Can you work these out from the model? Positions are in its coordinate system, mm. Face numbers are marked on the shaded views. A direction names the side the tool comes from. Give positions to 0.01 mm unless a question says otherwise; leave off trailing zeros. Write each loop counter-clockwise with the first axis right and the second up, starting at its lowest first coordinate (ties: lowest second). Pieces come first, ordered by that corner, then holes.
Autodesk Inventor part; units mm, degrees
ref_plane "YZ Plane" through (0, 0, 0) normal (1, 0, 0) x (0, 1, 0)
ref_plane "XZ Plane" through (0, 0, 0) normal (0, 1, 0) x (-1, 0, 0)
ref_plane "XY Plane" through (0, 0, 0) normal (0, 0, 1) x (1, 0, 0)
sketch "Skizze1" plane through (0, 0, 0) normal (0, 1, 0) x (-1, 0, 0)
  arc A0 (-8, 0) -> (8, 0) centre (0, 0) ccw
  line L0 (8, 0) -> (8, 11)
  line L1 (8, 17) -> (-8, 17)
  line L2 (-8, 17) -> (-8, 0)
  line L3 (8, 17) -> (19, 17)
  line L4 (19, 17) -> (19, 11)
  line L5 (19, 11) -> (8, 11)
  dimension "d0" = 16
  dimension "d1" = 16
  dimension "d2" = 6
  dimension "d3" = 19
  dimension "d4" = 11
  dimension "d5" = 17
extrude "Extrusion1" add sketch "Skizze1" along normal blind 50
sketch "Skizze2" plane through (0, 50, 0) normal (0, 1, 0) x (1, 0, 0)
  arc A0 (8, 0) -> (-8, 0) centre (0, 0) ccw
hole "Bohrung1" at (0, 50, 0) direction (0, -1, 0) diameter 6 end through all
sketch "Skizze3" plane through (-19, 0, 11) normal (-1, 0, 0) x (0, 0, 1)
  line L0 (0, 0) -> (0, 50)
  line L1 (0, 31) -> (-11, 31)
  arc A0 (-11, 31) -> (-11, 19) centre (-11, 25) ccw
  line L2 (-11, 19) -> (0, 19)
  line L3 (0, 31) -> (0, 19)
  point P0 (-11, 0)
  point P1 (0, 25)
  dimension "d15" = 6
extrude "Extrusion2" add sketch "Skizze3" against normal up to surface (11 mm away)
sketch "Skizze4" plane through (-19, 0, 11) normal (-1, 0, 0) x (0, 0, 1)
  arc A0 (-11, 31) -> (-11, 19) centre (-11, 25) ccw
  point P0 (-11, 0)
hole "Bohrung2" at (-19, 25, 0) direction (1, 0, 0) diameter 9 depth 11
sketch "Skizze5" plane through (-8, 50, 11) normal (0, 0, -1) x (-1, 0, 0)
  line L0 (11, -19) -> (11, 0)
  line L1 (11, -31) -> (11, -19)
  point P0 (-8, -50)
  point P1 (4.5, -12.5)
  point P2 (4.5, -37.5)
  point P3 (11, -25)
  dimension "d32" = 6.5
  dimension "d33" = 12.5
  dimension "d34" = 25
hole "Bohrung3" at (-12.5, 37.5, 11) at (-12.5, 12.5, 11) direction (0, 0, 1) diameter 4.134 end through all
properties part number "103"
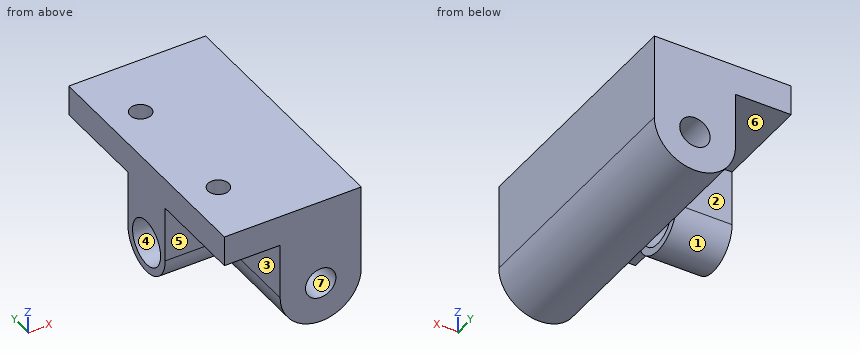
(1) Imagine slicing it at C-C, the plane z = 15.25. Write out the boundary of the cut face in (x, y).
Returned:
outline: (-19, 0) - (8, 0) - (8, 50) - (-19, 50) - close; hole circle Ø4.13 at (-12.5, 12.5); hole circle Ø4.13 at (-12.5, 37.5)
(2) If we mould it in two halves opening along Z, with no side actions, what happens to the marked faces 5, 6 and 7? For each: +Z half, -Z half, draft (parallel to the pull), parting line (faces both ways), or undercut.
Returned:
face 5: draft
face 6: -Z half
face 7: undercut
(3) Imagine slicing it at D-D, the plane y = 25. Write out the boundary of the cut face in (x, z), plus the area to 3 significant figures.
Returned:
outline: (-19, -6) - (-8, -6) - (-8, -4.5) - (-19, -4.5) - close; (-19, 4.5) - (-8, 4.5) - (-8, 0) arc R8 ccw to (8, 0) - (8, 17) - (-19, 17) - close; hole circle Ø6 at (0, 0)
area: 498 mm2
(4) If I drill on L1, parallel to Y at x = -12.5, z = 15.25; L2, parallel to Z at x = 0.25, y = 35.5; L3, parallel to Y at x = -13.5, z = 0, over which ranges is the centre line in solid material (lowest first)?
Returned:
L1: y = 0 to 10.43, 14.57 to 35.43, 39.57 to 50
L2: z = -8 to -2.99, 2.99 to 17
L3: y = 19 to 20.5, 29.5 to 31
(5) Imagine slicing it at A-A, the plane x = -12.5. Write out the boundary of the cut face in (y, z).
Returned:
outline: (0, 11) - (10.43, 11) - (10.43, 17) - (0, 17) - close; (14.57, 11) - (19, 11) - (19, 0) arc R6 ccw to (31, 0) - (31, 11) - (35.43, 11) - (35.43, 17) - (14.57, 17) - close; (39.57, 11) - (50, 11) - (50, 17) - (39.57, 17) - close; hole circle Ø9 at (25, 0)
(6) Will these pins go through, and if not, where does the flat tip stop? P1, Ø5.5, axis at x = -12, y = 36.5, coming from the -Z side; P2, Ø5.5, axis at x = -12, z = 4.5, coming from the +Y side; P3, Ø5.5, axis at x = -11.5, z = 8, coming from the -Y side.
Returned:
P1: stops at z = 11
P2: stops at y = 31
P3: stops at y = 19
(7) Imagine slicing it at B-B, the plane y = 12.5. Write out the boundary of the cut face in (x, z).
Returned:
outline: (-19, 11) - (-14.57, 11) - (-14.57, 17) - (-19, 17) - close; (-10.43, 11) - (-8, 11) - (-8, 0) arc R8 ccw to (8, 0) - (8, 17) - (-10.43, 17) - close; hole circle Ø6 at (0, 0)
(8) For the marked faces 1, 2, 3 and 4, which set-ups out of +Z, -Z, +X, -X, +Y, -Y let a thin tool reach every point of the face, with its end or its side?
Returned:
face 1: -Z, -X
face 2: -Z, -X, +Y
face 3: -Z, -X, -Y
face 4: -X
